Design review of the part built by this model. Coordinates are the model's own, in mm. A direction names the side the tool comes from. Coordinates: 2 decimals unless noted, no trailing zeros. Write each loop counter-clockwise with the first axis right and the second up, starting at its lowest first coordinate (ties: lowest second). Pieces come first, ordered by that corner, then holes. Notation, with made-up numbers: (13, 89.25) -> (31, 89.25) arc R23 cw to (31, 101.25) -> close; hole circle Ø6 at (24, 19.5). An arc over 180 degrees is marked (long way). Answer in a Markdown table with one row per item. Add a question column.
Item 1: Take a section at D-D, the plane x = -28. Write out the cut boundary in (y, z).
Item 2: Take a section at B-B, the plane y = 1. Write out the cut boundary in (x, z), and give its area (3 significant figures).
Item 3: Clearance check with flat-ended pins moving along their axes: P1, Ø1.8, axis at x = -26.26, y = 11.32, coming from the +Z side; P2, Ø1, axis at y = 5.5, z = 0.5, coming from the +X side. State where each tip first meets the part, or that it passes through.
Item 4: Draft analysis for pull direction Y (two halves, no side actions). For faces 3 (the face through (-13.135, 17.222, 0.986)), 4 (the face through (-30, 12.16, 0.99)), 5 (the face through (-6.824, 16.067, 0.986)), 6 (the face through (-27.05, 10.71, 0.99)), state which applies: released by +Y, released by -Y, zero draft, split by the parting line, or undercut.
Item 5: Take a section at C-C, the plane z = 1. Write out the cut boundary in (x, y) (3 decimals), and give its area (3 significant figures).
Item 6: For faces 1 (the face through (-22.36, 19.64, 0.99)), 2 (the face through (-10.5, 18.2, 1)), list the 3-axis set-ups (+Z, -Z, +X, -X, +Y, -Y) from which the entire face can be reached by the end or side of a thin tool; tool diameter is ignored.
Item 7: Take a section at A-A, the plane x = 0. Write out the cut boundary in (y, z), and give its area (3 significant figures).
Item 8: To check wall thickness, follow line 1 (Y direction, x = 0, z = 0.85); line 2 (Y direction, x = -24, z = 1.4); line 3 (X direction, y = 3, z = 0.3). State the ranges of each line that lie inside material, in increasing order.
from build123d import *

# Parameters (mm, degrees)
ESQUISSE1_R        = 4
ESQUISSE1_R_2      = 1
BOSS_EXTRU_1_DEPTH = 2
CONG_1_R           = 1
CONG_2_R           = 11


with BuildPart() as part:
    # Esquisse1 → Boss.-Extru.1 (new body)
    with BuildSketch(Plane.XY):
        with BuildLine():
            Line((-3.728432128, 14.529239273), (-10.902133324, 18.092613259))
            Line((-10.902133324, 18.092613259), (-9.77414371, 20.363455577))
            Line((-9.77414371, 20.363455577), (-25.005281494, 27.929179137))
            ThreePointArc((-25.005281494, 27.929179137), (-32.144223962, 28.809157948), (-34.856074883, 22.146971607))
            Line((-34.856074883, 22.146971607), (-25.005281494, 1.884444499))
            Line((-25.005281494, 1.884444499), (-9.850606554, -11.31218593))
            ThreePointArc((-9.850606554, -11.31218593), (-0.12474397, -14.999481289), (9.661100255, -11.47445606))
            ThreePointArc((9.661100255, -11.47445606), (9.328139992, -8.064479271), (12.711512496, -7.524484146))
            ThreePointArc((12.711512496, -7.524484146), (16.183775509, -6.191442889), (14.487891216, -2.881218443))
            ThreePointArc((14.487891216, -2.881218443), (12.323112571, -0.335609675), (14.623234656, 2.088401251))
            ThreePointArc((14.623234656, 2.088401251), (16.496773903, 5.301415429), (13.102212542, 6.821468911))
            ThreePointArc((13.102212542, 6.821468911), (9.820570557, 7.451720018), (10.097110191, 10.781872629))
            ThreePointArc((10.097110191, 10.781872629), (9.547104174, 14.460337363), (5.948313856, 13.521019705))
            ThreePointArc((5.948313856, 13.521019705), (2.883768887, 11.988907316), (1.167882396, 14.954465912))
            ThreePointArc((1.167882396, 14.954465912), (-1.297808983, 14.94375093), (-3.728432128, 14.529239273))
        make_face()
        with Locations((-20.325227829, 4.439090716)):
            Circle(ESQUISSE1_R, mode=Mode.SUBTRACT)
        with Locations((-26.256387143, 11.319323515)):
            Circle(ESQUISSE1_R_2, mode=Mode.SUBTRACT)
        with BuildLine():
            ThreePointArc((-29.058075564, 23.063121212), (-29.928943128, 25.754141406), (-27.237922934, 26.625008971))
            Line((-27.237922934, 26.625008971), (-14.025891569, 19.873557138))
            ThreePointArc((-14.025891569, 19.873557138), (-13.155024005, 17.182536944), (-15.846044199, 16.31166938))
            Line((-15.846044199, 16.31166938), (-29.058075564, 23.063121212))
        make_face(mode=Mode.SUBTRACT)
        Circle(ESQUISSE1_R, mode=Mode.SUBTRACT)
    extrude(amount=BOSS_EXTRU_1_DEPTH)

    # Congé1
    cong_1_edges = [part.edges().sort_by_distance(p)[0] for p in [
        (-9.77414371, 20.363455577, 1),
        (-10.902133324, 18.092613259, 1),
    ]]
    fillet(cong_1_edges, radius=CONG_1_R)

    # Congé2
    cong_2_edges = [part.edges().sort_by_distance(p)[0] for p in [
        (-25.005281494, 27.929179137, 1),
    ]]
    fillet(cong_2_edges, radius=CONG_2_R)


solid = part.part
Answers:
| question | item | result |
|---|---|---|
| 1 | outline | (8.04, 0) -> (22.52, 0) -> (22.52, 2) -> (8.04, 2) -> close; (26.84, 0) -> (29.51, 0) -> (29.51, 2) -> (26.84, 2) -> close |
| 2 | outline | (-23.99, 0) -> (-22.37, 0) -> (-22.37, 2) -> (-23.99, 2) -> close; (-18.28, 0) -> (-3.87, 0) -> (-3.87, 2) -> (-18.28, 2) -> close; (3.87, 0) -> (12.75, 0) -> (12.75, 2) -> (3.87, 2) -> close |
| 2 | area | 49.8 mm^2 |
| 3 | P1 | passes through |
| 3 | P2 | stops at x = 16.57 |
| 4 | face 3 | undercut |
| 4 | face 4 | released by -Y |
| 4 | face 5 | released by +Y |
| 4 | face 6 | undercut |
| 5 | outline | (-34.856, 22.147) -> (-25.005, 1.884) -> (-9.851, -11.312) arc R15 ccw to (9.661, -11.474) arc R2.5 cw to (12.712, -7.524) arc R2.5 ccw (long way) to (14.488, -2.881) arc R2.5 cw to (14.623, 2.088) arc R2.5 ccw (long way) to (13.102, 6.821) arc R2.5 cw to (10.097, 10.782) arc R2.5 ccw (long way) to (5.948, 13.521) arc R2.5 cw to (1.168, 14.954) arc R15 ccw to (-3.728, 14.529) -> (-10.007, 17.648) arc R1 cw to (-10.457, 18.988) -> (-10.219, 19.468) arc R1 ccw to (-10.67, 20.808) -> (-23.848, 27.354) arc R11 cw to (-25.584, 28.428) arc R5.916 ccw to start; hole (-29.058, 23.063) -> (-15.846, 16.312) arc R2 ccw to (-14.026, 19.874) -> (-27.238, 26.625) arc R2 ccw to start; hole circle Ø2 at (-26.256, 11.319); hole circle Ø8 at (-20.325, 4.439); hole circle Ø8 at (0, 0) |
| 5 | area | 1,060 mm^2 |
| 6 | face 1 | +Z, -Z |
| 6 | face 2 | +Z, -Z, +X |
| 7 | outline | (-15, 0) -> (-4, 0) -> (-4, 2) -> (-15, 2) -> close; (4, 0) -> (15, 0) -> (15, 2) -> (4, 2) -> close |
| 7 | area | 44.0 mm^2 |
| 8 | line 1 | y = -15 to -4, 4 to 15 |
| 8 | line 2 | y = 1.01 to 2.86, 6.02 to 20.48, 24.97 to 27.43 |
| 8 | line 3 | x = -25.55 to -24.06, -16.59 to -2.65, 2.65 to 16.09 |
